```python
from build123d import *

# Parameters (mm, degrees)
SKETCH1_R           = 3.75
BOSS_EXTRUDE1_DEPTH = 9.525
SKETCH2_R           = 6.35
CUT_EXTRUDE1_DEPTH  = 10.525


with BuildPart() as part:
    # Sketch1 → Boss-Extrude1 (new body)
    with BuildSketch(Plane.XY):
        Polygon((40.03500006, -9.525), (7.01500006, -9.525), (7.01500006, 0), (0, 0), (0, -33.02), (9.525, -33.02), (9.525, -66.04), (0, -66.04), (0, -99.06), (9.525, -99.06), (9.525, -132.08), (0, -132.08), (0, -165.1), (47.05000012, -165.1), (47.05000012, -132.08), (37.52500012, -132.08), (37.52500012, -99.06), (47.05000012, -99.06), (47.05000012, -66.04), (37.52500012, -66.04), (37.52500012, -33.02), (47.05000012, -33.02), (47.05000012, 0), (40.03500006, 0), align=None)
        with Locations((23.52500006, -23.525)):
            Circle(SKETCH1_R, mode=Mode.SUBTRACT)
    extrude(amount=BOSS_EXTRUDE1_DEPTH)

    # Sketch2 → Cut-Extrude1 (cut, through all)
    with BuildSketch(Plane.XY.offset(9.525)):
        with Locations((23.52500006, -148.59)):
            Circle(SKETCH2_R)
    extrude(amount=-CUT_EXTRUDE1_DEPTH, mode=Mode.SUBTRACT)


solid = part.part
```
Geometry check sheet. Reference: the model listing, model coordinates, mm. A direction names the side the tool comes from. Give positions to 0.01 mm unless a question says otherwise; leave off trailing zeros. Order: outer loops, then holes, each group sorted by start corner. A loop starts at its lowest first (then second) coordinate and runs counter-clockwise, first axis right, second up. Notation, with made-up numbers: (7.25, 23.25) - (28.25, 23.25) arc R10 cw to (28.25, 28.25) - close; hole circle Ø8 at (62, 85.25). An arc over 180 degrees is marked (long way). Answer in a Markdown table with one row per item. Add a question column.
Q1. Tool access check on faces 1 (the flat face through (47.05, -149, 5)), 2 (the flat face through (37.525, -116, 5)), 3 (the flat face through (40.035, -5, 5)), 4 (the flat face through (5, -132.08, 5)). Record the directions out of +Z, -Z, +X, -X, +Y, -Y that give a thin tool (end or side, any length) a straight path to the whole face; none if there is none.
Q2. Cross-section at D-D, the plane x = 23. Enter the section's corners in (y, z) (3 decimals).
Q3. Cross-section at C-C, the plane z = 3.25. Enter the section's corners in (x, y) (3 decimals).
Q4. Gauge pin test, flat ends, axial feed: pin 1 (3 mm diameter, centred on y = -45, z = 5.5, fed in from -X) (3 decimals); pin 2 (1 mm diameter, centred on y = -65, z = 5.5, fed in from +X) (3 decimals); pin 3 (5 mm diameter, centred on x = 29, z = 2.5, fed in from +Y) (3 decimals); pin 4 (11.5 mm diameter, centred on x = 23.525, y = -148.59, fed in from +Z). Record the tip position at first contact, or that the pin passes through.
Q5. Cross-section at B-B, the plane x = 41.5. Enter the section's corners in (y, z) (3 decimals).
Q6. Cross-section at A-A, the plane y = -148.59. Enter the section's corners in (x, z) (3 decimals), then the cut area to 3 significant figures.
Q7. Mould release check, pull along Y, two halves, no side actions. Record for faces 5 (the flat face through (47.05, -83, 5)), 6 (the flat face through (9.525, -49, 5)), 7 (the flat face through (4, 0, 5)), 8 (the flat face through (5, -33.02, 5)): pulls with the +Y half, pulls with the -Y half, needs draft (parallel to the pull), parting line crosses it, or undercut.
Q8. Material ranges on probe 1 along Y at (x, z) = (2.5, 5.5); probe 2 along Y at (x, z) = (8.5, 1.25) (3 decimals); probe 3 along Y at (x, z) = (14.5, 4.5) (3 decimals), recorded low to high. Write a range as from..to.
Check values:
| question | item | result |
|---|---|---|
| 1 | face 1 | +Z, -Z, +X, +Y, -Y |
| 1 | face 2 | +Z, -Z, +X |
| 1 | face 3 | +Z, -Z, +Y |
| 1 | face 4 | +Z, -Z, -X |
| 2 | outline | (-165.1, 0) - (-154.918, 0) - (-154.918, 9.525) - (-165.1, 9.525) - close; (-142.262, 0) - (-27.238, 0) - (-27.238, 9.525) - (-142.262, 9.525) - close; (-19.812, 0) - (-9.525, 0) - (-9.525, 9.525) - (-19.812, 9.525) - close |
| 3 | outline | (0, -165.1) - (47.05, -165.1) - (47.05, -132.08) - (37.525, -132.08) - (37.525, -99.06) - (47.05, -99.06) - (47.05, -66.04) - (37.525, -66.04) - (37.525, -33.02) - (47.05, -33.02) - (47.05, 0) - (40.035, 0) - (40.035, -9.525) - (7.015, -9.525) - (7.015, 0) - (0, 0) - (0, -33.02) - (9.525, -33.02) - (9.525, -66.04) - (0, -66.04) - (0, -99.06) - (9.525, -99.06) - (9.525, -132.08) - (0, -132.08) - close; hole circle Ø12.7 at (23.525, -148.59); hole circle Ø7.5 at (23.525, -23.525) |
| 4 | pin 1 | stops at x = 9.525 |
| 4 | pin 2 | stops at x = 37.525 |
| 4 | pin 3 | stops at y = -9.525 |
| 4 | pin 4 | passes through |
| 5 | outline | (-165.1, 0) - (-132.08, 0) - (-132.08, 9.525) - (-165.1, 9.525) - close; (-99.06, 0) - (-66.04, 0) - (-66.04, 9.525) - (-99.06, 9.525) - close; (-33.02, 0) - (0, 0) - (0, 9.525) - (-33.02, 9.525) - close |
| 6 | outline | (0, 0) - (17.175, 0) - (17.175, 9.525) - (0, 9.525) - close; (29.875, 0) - (47.05, 0) - (47.05, 9.525) - (29.875, 9.525) - close |
| 6 | area | 327 mm^2 |
| 7 | face 5 | needs draft |
| 7 | face 6 | undercut |
| 7 | face 7 | pulls with the +Y half |
| 7 | face 8 | undercut |
| 8 | probe 1 | y = -165.1..-132.08, -99.06..-66.04, -33.02..0 |
| 8 | probe 2 | y = -165.1..-132.08, -99.06..-66.04, -33.02..-9.525 |
| 8 | probe 3 | y = -165.1..-9.525 |
